Verification items for the finished model (mm, model axes). Face numbers are marked on the shaded views. Give positions to 0.01 mm unless a question says otherwise; leave off trailing zeros. Loops run counter-clockwise (first coordinate to the right, second up) from the corner with the lowest first, then second, coordinate; pieces in that order, holes last. Notation, with made-up numbers: M 82,88 L 111,88 A17 ccw 111,117 Z; hole C 47.25,-39.5 d6. An arc over 180 degrees is marked long. Use a Markdown table: item, result.
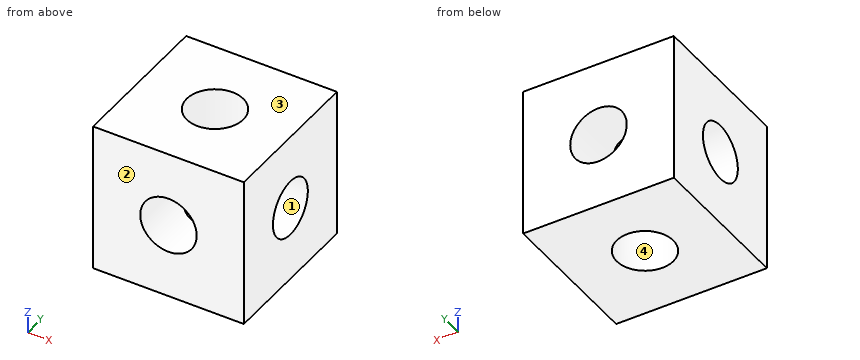
Autodesk Inventor part; units mm, degrees
ref_plane "YZ Plane" through (0, 0, 0) normal (1, 0, 0) x (0, 1, 0)
ref_plane "XZ Plane" through (0, 0, 0) normal (0, 1, 0) x (-1, 0, 0)
ref_plane "XY Plane" through (0, 0, 0) normal (0, 0, 1) x (1, 0, 0)
sketch "草图1" plane through (0, 0, 0) normal (0, 0, 1) x (1, 0, 0)
  line L0 (4, -4) -> (-4, -4)
  line L1 (-4, -4) -> (-4, 4)
  line L2 (-4, 4) -> (4, 4)
  line L3 (4, 4) -> (4, -4)
  line L4 (4, -4) -> (-4, 4) construction
  line L5 (-4, -4) -> (4, 4) construction
  point P0 (0, 0)
  dimension "d0" = 8
  dimension "d1" = 8
extrude "拉伸1" add sketch "草图1" along normal blind 8
sketch "草图2" plane through (-4, -4, 0) normal (0, -1, 0) x (1, 0, 0)
  line L0 (8, 8) -> (0, 8)
  line L1 (0, 8) -> (8, 0)
  circle A0 centre (4, 4) radius 1.5
  point P0 (4, 0)
  dimension "d4" = 3
extrude "拉伸2" cut sketch "草图2" against normal blind 8
sketch "草图3" plane through (0, 0, 0) normal (0, 0, -1) x (-1, 0, 0)
  circle A0 centre (0, 0) radius 1.5
  dimension "d7" = 3
extrude "拉伸3" cut sketch "草图3" against normal blind 8
sketch "草图4" plane through (4, -4, 0) normal (1, 0, 0) x (0, 0, -1)
  line L0 (0, 8) -> (0, 0)
  line L1 (0, 8) -> (-8, 0)
  circle A0 centre (-4, 4) radius 1.5
  point P0 (0, 4)
  dimension "d10" = 3
extrude "拉伸4" cut sketch "草图4" against normal blind 14.25
properties part number "8X"
(1) Material ranges on line 1 (Z direction, x = -2.65, y = 0); line 2 (X direction, y = -3.5, z = 4); line 3 (X direction, y = 0.75, z = 1.75), recorded low to high.
Results below:
| item | result |
|---|---|
| line 1 | 0 to 2.5, 5.5 to 8 |
| line 2 | -4 to -1.5, 1.5 to 4 |
| line 3 | -4 to -1.3, 1.3 to 4 |
(2) Cross-section at D-D on z = 1. Record the cut outline in (x, y).
Results below:
| item | result |
|---|---|
| outline | M -4,-4 L 4,-4 L 4,4 L -4,4 Z; hole C 0,0 d3 |
(3) Draft check along Y on the marked faces 1, 2, 3 and 4. Enter one of: +Y half, -Y half, draft (parallel to the pull), parting line (faces both ways), or undercut.
Results below:
| item | result |
|---|---|
| face 1 | undercut |
| face 2 | -Y half |
| face 3 | draft |
| face 4 | undercut |
(4) Gauge pin test, flat end, axial feed: P1, Ø4, axis at x = 0, z = 4, coming from the +Y side. Record the tip position at first contact, or that the pin passes through.
Results below:
| item | result |
|---|---|
| P1 | y = 4 |
(5) Cross-section at C-C on x = 2. Record the cut outline in (y, z), then the cut area to 3 significant figures.
Results below:
| item | result |
|---|---|
| outline | M -4,0 L 4,0 L 4,8 L -4,8 Z; hole C 0,4 d3 |
| area | 56.9 mm^2 |
(6) Cross-section at A-A on x = 0. Record the cut outline in (y, z), then the cut area to 3 significant figures.
Results below:
| item | result |
|---|---|
| outline | M -4,0 L -1.5,0 L -1.5,2.5 L -4,2.5 Z; M -4,5.5 L -1.5,5.5 L -1.5,8 L -4,8 Z; M 1.5,0 L 4,0 L 4,2.5 L 1.5,2.5 Z; M 1.5,5.5 L 4,5.5 L 4,8 L 1.5,8 Z |
| area | 25.0 mm^2 |
